Autodesk Inventor part; units mm, degrees
ref_plane "YZ Plane" through (0, 0, 0) normal (1, 0, 0) x (0, 1, 0)
ref_plane "XZ Plane" through (0, 0, 0) normal (0, 1, 0) x (-1, 0, 0)
ref_plane "XY Plane" through (0, 0, 0) normal (0, 0, 1) x (1, 0, 0)
sketch "Sketch1" plane through (0, 0, 0) normal (0, 1, 0) x (-1, 0, 0)
  line L0 (0, 0) -> (70, 0)
  line L1 (70, 0) -> (70, -50)
  line L2 (70, -50) -> (0, -50)
  line L3 (0, -50) -> (0, 0)
  dimension "d0" = 70
  dimension "d1" = 50
extrude "Extrusion1" add sketch "Sketch1" along normal blind 2
sketch "Sketch2" plane through (0, 2, 0) normal (0, 1, 0) x (1, 0, 0)
  line L0 (-70, 50) -> (-70, 0)
  line L1 (-70, 25) -> (-60, 25)
  line L2 (-60, 25) -> (-60, 15)
  line L3 (-60, 15) -> (-10, 15)
  line L4 (-10, 15) -> (-10, 35)
  line L5 (-10, 35) -> (-60, 35)
  line L6 (-60, 35) -> (-60, 15)
  point P0 (0, 0)
  dimension "d4" = 10
  dimension "d5" = 10
  dimension "d6" = 50
  dimension "d7" = 20
  dimension "d20" = 25
  dimension "d21" = 25
extrude "Extrusion2" add sketch "Sketch2" along normal blind 15
sketch "Sketch3" plane through (0, 2, 0) normal (0, 1, 0) x (1, 0, 0)
  line L0 (0, 50) -> (-70, 50)
  line L1 (0, 50) -> (-30, 50)
  line L2 (-30, 50) -> (-30, 45)
  line L3 (-30, 45) -> (0, 45)
  line L4 (0, 45) -> (0, 50)
  line L5 (-70, 50) -> (-70, 0)
  line L6 (-70, 0) -> (-40, 0)
  line L7 (-40, 0) -> (-40, 5)
  line L8 (-40, 5) -> (-70, 5)
  line L9 (-70, 5) -> (-70, 0)
  line L10 (-30, 45) -> (-40, 45)
  line L11 (-40, 45) -> (-40, 5)
  line L12 (-40, 5) -> (-30, 5)
  line L13 (-30, 5) -> (-30, 45)
  circle A0 centre (-30, 5) radius 0.5
  circle A1 centre (-40, 5) radius 0.5
  circle A2 centre (-30, 45) radius 0.5
  circle A3 centre (-40, 45) radius 0.5
  point P0 (0, 0)
  dimension "d10" = 30
  dimension "d11" = 5
  dimension "d12" = 30
  dimension "d13" = 5
  dimension "d14" = 1
  dimension "d15" = 1
  dimension "d16" = 1
  dimension "d17" = 1
extrude "Extrusion3" cut sketch "Sketch3" against normal blind 15 contours A2 L3 L2 | L2 L10 A2 | A2 L13 L3 | L13 A2 L10 | A1 L11 L8 | L8 L7 A1 | A3 L11 L10 | L10 L11 A3 | A0 L12 L13 | L13 L12 A0 | L12 A1 L7 | L11 A1 L12
sketch "Sketch4" plane through (0, 2, 0) normal (0, 1, 0) x (1, 0, 0)
  line L0 (0, 0) -> (0, 50)
  line L1 (-70, 50) -> (-70, 0)
  line L2 (0, 0) -> (-70, 0)
  line L3 (-70, 0) -> (-70, 15)
  line L4 (-70, 15) -> (0, 15)
  line L5 (0, 15) -> (0, 0)
  dimension "d22" = 15
extrude "Extrusion4" cut sketch "Sketch4" against normal blind 15
properties part number "RPpico_dummy"
Geometry check sheet. Reference: the model listing, model coordinates, mm. A direction names the side the tool comes from. Round coordinates to 2 decimals unless told otherwise and drop trailing zeros. Write each loop counter-clockwise with the first axis right and the second up, starting at its lowest first coordinate (ties: lowest second). Pieces come first, ordered by that corner, then holes. Notation, with made-up numbers: (29.5, 15) - (35.5, 15) arc R22 cw to (35.5, 27) - close; hole circle Ø3 at (64, 27). An arc over 180 degrees is marked (long way). One line per item, written item: value.
1. Cross-section at B-B on x = -41.5. Record the boundary of the cut face in (y, z).
The answers:
outline: (0, -50) - (2, -50) - (2, -35) - (17, -35) - (17, -15) - (0, -15) - close
2. Scan lines: L1, parallel to X at y = 1.5, z = -45; L2, parallel to Z at x = -40, y = 0.9; L3, parallel to Y at x = -11.5, z = -48. Record each from-to range of solid material in increasing order.
The answers:
L1: x = -70 to -40.5, -39.5 to -30.5, -29.5 to 0
L2: z = -50 to -45.5, -44.5 to -15
L3: y = 0 to 2
3. Cross-section at D-D on z = -47. Record the boundary of the cut face in (x, y).
The answers:
outline: (-70, 0) - (0, 0) - (0, 2) - (-70, 2) - close
4. Set-up check for faces 1 (the face through (-35, 9, -35)), 2 (the face through (-10, 9, -25)), 3 (the face through (-60, 9, -25)): record each of +Z, -Z, +X, -X, +Y, -Y from which the full face is reachable in a straight line by a thin tool's end or side.
The answers:
face 1: -Z, +X, -X, +Y
face 2: +Z, -Z, +X, +Y
face 3: +Z, -Z, -X, +Y
5. Cross-section at C-C on y = 6.75. Record the boundary of the cut face in (x, z), and give its area (3 significant figures).
The answers:
outline: (-60, -35) - (-10, -35) - (-10, -15) - (-60, -15) - close
area: 1,000 mm^2
6. Depth check by flat-ended pin: pin 1 Ø1.5 at (y, z) = (8.5, -23.5) entering from -X; pin 2 Ø5 at (x, z) = (-25.5, -25.5) entering from -Y; pin 3 Ø6 at (x, z) = (-10, -40.5) entering from +Y; pin 4 Ø7.5 at (y, z) = (11.5, -29) entering from +X. Enter the tip coordinate at first touch or a pass-through.
The answers:
pin 1: stops at x = -60
pin 2: stops at y = 0
pin 3: stops at y = 2
pin 4: stops at x = -10
7. Cross-section at A-A on z = -28. Record the boundary of the cut face in (x, y).
The answers:
outline: (-70, 0) - (0, 0) - (0, 2) - (-10, 2) - (-10, 17) - (-60, 17) - (-60, 2) - (-70, 2) - close
